from build123d import *

# Parameters (mm, degrees)
SKETCH_1_R          = 3.5
EXTRUDE_1_DEPTH     = 2
SKETCH_2_R          = 2
EXTRUDE_2_DEPTH     = 12
CUT_EXTRUDE_START   = -3
SKETCH_3_R          = 2
SKETCH_3_R_2        = 1.5
CUT_EXTRUDE_1_DEPTH = 0.6
CHAMFER_1_SIZE      = 0.5
FILLET_1_R          = 0.4


with BuildPart() as part:
    # 草图1 → 凸台-拉伸1 (new body)
    with BuildSketch(Plane.XY):
        Circle(SKETCH_1_R)
    extrude(amount=EXTRUDE_1_DEPTH)

    # 草图2 → 凸台-拉伸2 (add)
    with BuildSketch(Plane.XY.offset(2)):
        Circle(SKETCH_2_R)
    extrude(amount=EXTRUDE_2_DEPTH)

    # 草图3 → 切除-拉伸1 (cut)
    with BuildSketch(Plane.XY.offset(14).offset(CUT_EXTRUDE_START)):
        Circle(SKETCH_3_R)
        Circle(SKETCH_3_R_2, mode=Mode.SUBTRACT)
    extrude(amount=CUT_EXTRUDE_1_DEPTH, mode=Mode.SUBTRACT)

    # 倒角1
    chamfer_1_edges = [part.edges().sort_by_distance(p)[0] for p in [
        (-2, 0, 14),
    ]]
    chamfer(chamfer_1_edges, length=CHAMFER_1_SIZE)

    # 圆角1
    fillet_1_edges = [part.edges().sort_by_distance(p)[0] for p in [
        (-3.5, 0, 0),
        (-3.5, 0, 2),
    ]]
    fillet(fillet_1_edges, radius=FILLET_1_R)


solid = part.part
Can you work these out from the model? Positions are in its coordinate system, mm. A direction names the side the tool comes from. Round coordinates to 2 decimals unless told otherwise and drop trailing zeros. Loops run counter-clockwise (first coordinate to the right, second up) from the corner with the lowest first, then second, coordinate; pieces in that order, holes last. Notation, with made-up numbers: (17, 9) - (26, 9) arc R21 cw to (26, 47) - close; hole circle Ø10 at (71.25, -9.75). An arc over 180 degrees is marked (long way). Answer in a Markdown table with one row per item. Add a question column.
Q1. Which directions (+Z, -Z, +X, -X, +Y, -Y) give clear straight access to the entire face, cutting with the end or side of a thin tool? Please do faces 1 (the flat face through (0, 0, 14)), 2 (the flat face through (2, -1, 2)).
Q2. I need wall thicknesses on L1, parallel to Z at x = -3, y = -0.75; L2, parallel to Z at x = -1.5, y = 1; L3, parallel to Y at x = 0, z = 7.25. Which ranges of each line are inside material? Lowest first, please.
Q3. We'd pull the mould along Z, two halves only. Please class faces 3 (the cylindrical face through (0, -2, 13)), 4 (the cylindrical face through (-1.5, 0.07, 11.3)), 5 (the flat face through (0, 0, 0)): pulls with the +Z half, pulls with the -Z half, needs draft (parallel to the pull), parting line crosses it, or undercut.
Q4. I want a section at A-A on x = 0. List the corners of the cut face in (y, z) for me, and give its area (3 significant figures).
Q5. I want a section at D-D on z = 4. List the corners of the cut face in (x, y) for me, and give its area (3 significant figures).
Q6. For pin 1 Ø1.5 at (x, y) = (-1.5, -2.5) entering from +Z; pin 2 Ø2 at (y, z) = (-2.5, 12.5) entering from +X; pin 3 Ø3 at (y, z) = (-1, 8.5) entering from +X, each with a flat end and sliding along its axis, tell me the tip position at first contact or that it passes through.
Q7. I want a section at C-C on z = 1. List the corners of the cut face in (x, y) for me.
A:
| question | item | result |
|---|---|---|
| 1 | face 1 | +Z, +X, -X, +Y, -Y |
| 1 | face 2 | +Z |
| 2 | L1 | 0 to 2 |
| 2 | L2 | 0 to 11, 11.6 to 13.7 |
| 2 | L3 | -2 to 2 |
| 3 | face 3 | needs draft |
| 3 | face 4 | undercut |
| 3 | face 5 | pulls with the -Z half |
| 4 | outline | (-3.5, 0.4) arc R0.4 ccw to (-3.1, 0) - (3.1, 0) arc R0.4 ccw to (3.5, 0.4) - (3.5, 1.6) arc R0.4 ccw to (3.1, 2) - (2, 2) - (2, 11) - (1.5, 11) - (1.5, 11.6) - (2, 11.6) - (2, 13.5) - (1.5, 14) - (-1.5, 14) - (-2, 13.5) - (-2, 11.6) - (-1.5, 11.6) - (-1.5, 11) - (-2, 11) - (-2, 2) - (-3.1, 2) arc R0.4 ccw to (-3.5, 1.6) - close |
| 4 | area | 61.0 mm^2 |
| 5 | outline | circle Ø4 at (0, 0) |
| 5 | area | 12.6 mm^2 |
| 6 | pin 1 | z = 2 |
| 6 | pin 2 | x = 1.32 |
| 6 | pin 3 | x = 2 |
| 7 | outline | circle Ø7 at (0, 0) |
